Geometry check sheet. Reference: the model listing, model coordinates, mm. Give positions to 0.01 mm unless a question says otherwise; leave off trailing zeros. Loops run counter-clockwise (first coordinate to the right, second up) from the corner with the lowest first, then second, coordinate; pieces in that order, holes last. Notation, with made-up numbers: (-30.75, 0) -> (-9.75, 0) arc R24 ccw to (-9.75, 20) -> close; hole circle Ø11 at (-20, 30). An arc over 180 degrees is marked (long way). Write item = value, one per line. Start each with the question number.
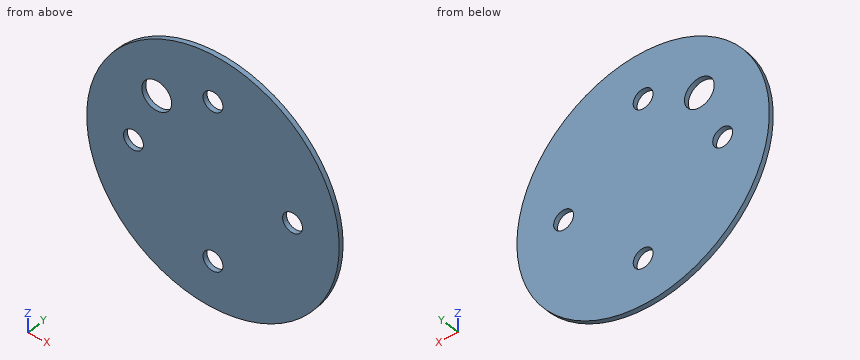
```python
from build123d import *

# Parameters (mm, degrees)
F0_R     = 127
F0_R_2   = 10
F0_R_3   = 15
F1_DEPTH = 4.763


with BuildPart() as f1:
    # F0 (on Front) → F1 (new body)
    with BuildSketch(Plane.XZ):
        Circle(F0_R)
        with Locations((0, -80)):
            Circle(F0_R_2, mode=Mode.SUBTRACT)
        with Locations((-80, 0)):
            Circle(F0_R_2, mode=Mode.SUBTRACT)
        with Locations((-56.568542, 56.568542)):
            Circle(F0_R_3, mode=Mode.SUBTRACT)
        with Locations((80, 0)):
            Circle(F0_R_2, mode=Mode.SUBTRACT)
        with Locations((0, 80)):
            Circle(F0_R_2, mode=Mode.SUBTRACT)
    extrude(amount=F1_DEPTH)


solid = f1.part
```
1) Section check A-A (z = 87). Enter the section's corners in (x, y), plus the area to 3 significant figures.
2) Section check C-C (z = -5.5). Enter the section's corners in (x, y).
3) Section check B-B (x = -65.5). Enter the section's corners in (y, z), plus the area to 3 significant figures.
4) Section check D-D (y = -1.1). Enter the section's corners in (x, z), plus the area to 3 significant figures.
5) Depth check by flat-ended pin: pin 1 Ø2 at (y, z) = (-3.5, 55) entering from +X; pin 2 Ø2 at (y, z) = (-1, 81) entering from +X. Enter the tip coordinate at first touch or a pass-through.
6) Thickness scan on line 1 (Z direction, x = 0, y = -3.35); line 2 (Z direction, x = -47.5, y = -1.65); line 3 (Z direction, x = 80, y = -2.7). Record the ranges inside material, lowest first.
Check result:
q1.outline = (-92.52, -4.76) -> (-7.14, -4.76) -> (-7.14, 0) -> (-92.52, 0) -> close; (7.14, -4.76) -> (92.52, -4.76) -> (92.52, 0) -> (7.14, 0) -> close
q1.area = 813 mm2
q2.outline = (-126.88, -4.76) -> (-88.35, -4.76) -> (-88.35, 0) -> (-126.88, 0) -> close; (-71.65, -4.76) -> (71.65, -4.76) -> (71.65, 0) -> (-71.65, 0) -> close; (88.35, -4.76) -> (126.88, -4.76) -> (126.88, 0) -> (88.35, 0) -> close
q3.outline = (-4.76, -108.81) -> (0, -108.81) -> (0, 44.52) -> (-4.76, 44.52) -> close; (-4.76, 68.62) -> (0, 68.62) -> (0, 108.81) -> (-4.76, 108.81) -> close
q3.area = 922 mm2
q4.outline = circle Ø254 at (0, 0); hole circle Ø20 at (-80, 0); hole circle Ø30 at (-56.57, 56.57); hole circle Ø20 at (0, -80); hole circle Ø20 at (0, 80); hole circle Ø20 at (80, 0)
q4.area = 48,700 mm2
q5.pin_1 = 114.95
q5.pin_2 = 98.64
q6.line_1 = -127 to -90, -70 to 70, 90 to 127
q6.line_2 = -117.78 to 44.62, 68.52 to 117.78
q6.line_3 = -98.64 to -10, 10 to 98.64
